from build123d import *

# Parameters (mm, degrees)
F0_R     = 3.175
F1_DEPTH = 3.048


with BuildPart() as f1:
    # F0 (on Front) → F1 (new body)
    with BuildSketch(Plane.XZ):
        with BuildLine():
            ThreePointArc((9.4772553384, -0.9525), (9.5130563464, -0.4768479324), (9.525, 0))
            ThreePointArc((9.525, 0), (6.8544082857, 6.6138273378), (0.3401785714, 9.5189234444))
            ThreePointArc((0.3401785714, 9.5189234444), (-6.948684782, 6.5147068085), (-9.4772553384, -0.9525))
            ThreePointArc((-9.4772553384, -0.9525), (-6.2623833552, -7.1769199322), (0.3401786416, -9.5189234418))
            ThreePointArc((0.3401786416, -9.5189234418), (6.5147068341, -6.948684758), (9.4772553384, -0.9525))
        make_face()
        Circle(F0_R, mode=Mode.SUBTRACT)
        with BuildLine():
            ThreePointArc((0.3401785714, 9.5189234444), (6.8544082857, 6.6138273378), (9.525, 0))
            ThreePointArc((9.525, 0), (9.5130563464, -0.4768479324), (9.4772553384, -0.9525))
            Line((9.4772553384, -0.9525), (10.4932062399, 9.1560838367))
            Line((10.4932062399, 9.1560838367), (0.3401785714, 9.5189234444))
        make_face()
        with BuildLine():
            ThreePointArc((-9.4772553384, -0.9525), (-6.948684782, 6.5147068085), (0.3401785714, 9.5189234444))
            Line((0.3401785714, 9.5189234444), (10.4932062399, 9.1560838367))
            Line((10.4932062399, 9.1560838367), (15.7954255641, 61.9125))
            ThreePointArc((15.7954255641, 61.9125), (0, 47.625), (-15.7954255641, 61.9125))
            Line((-15.7954255641, 61.9125), (-9.4772553384, -0.9525))
        make_face()
        Polygon((4.1081828244, 15.4546830389), (2.8649913232, 15.4546830389), (1.5788532065, 18.7389689503), (-2.5598443184, 18.7389689503), (-3.8301599978, 15.4546830389), (-5.0462273207, 15.4546830389), (-0.9640385005, 25.825160507), (0.0463371378, 25.825160507), align=None, mode=Mode.SUBTRACT)
        Polygon((4.1081828244, 35.1287536323), (2.8649913232, 35.1287536323), (1.5788532065, 38.4130395436), (-2.5598443184, 38.4130395436), (-3.8301599978, 35.1287536323), (-5.0462273207, 35.1287536323), (-0.9640385005, 45.4992311004), (0.0463371378, 45.4992311004), align=None, mode=Mode.SUBTRACT)
        with BuildLine():
            Line((10.4932062399, 9.1560838367), (9.4772553384, -0.9525))
            ThreePointArc((9.4772553384, -0.9525), (6.5147068341, -6.948684758), (0.3401786416, -9.5189234418))
            Line((0.3401786416, -9.5189234418), (44.7334821429, -7.9324362036))
            ThreePointArc((44.7334821429, -7.9324362036), (36.5125, 0), (44.7334821429, 7.9324362036))
            Line((44.7334821429, 7.9324362036), (10.4932062399, 9.1560838367))
        make_face()
        with BuildLine():
            ThreePointArc((-15.7504882737, 65.484375), (-15.8737438155, 63.6997054867), (-15.7954255641, 61.9125))
            ThreePointArc((-15.7954255641, 61.9125), (0, 47.625), (15.7954255641, 61.9125))
            ThreePointArc((15.7954255641, 61.9125), (15.8550939106, 62.7052534459), (15.875, 63.5))
            ThreePointArc((15.875, 63.5), (15.8438414904, 64.4941387366), (15.7504882737, 65.484375))
            ThreePointArc((15.7504882737, 65.484375), (0, 79.375), (-15.7504882737, 65.484375))
        make_face()
        with Locations((0, 63.5)):
            Circle(F0_R, mode=Mode.SUBTRACT)
        with BuildLine():
            ThreePointArc((52.3875, 0), (50.1620069047, 5.5115227815), (44.7334821429, 7.9324362036))
            ThreePointArc((44.7334821429, 7.9324362036), (36.5125, 0), (44.7334821429, -7.9324362036))
            ThreePointArc((44.7334821429, -7.9324362036), (50.1620069047, -5.5115227815), (52.3875, 0))
        make_face()
        with Locations((44.45, 0)):
            Circle(F0_R, mode=Mode.SUBTRACT)
        with BuildLine():
            Line((-9.4502929642, 115.490625), (-15.7504882737, 65.484375))
            ThreePointArc((-15.7504882737, 65.484375), (0, 79.375), (15.7504882737, 65.484375))
            Line((15.7504882737, 65.484375), (9.4502929642, 115.490625))
            ThreePointArc((9.4502929642, 115.490625), (9.5063048942, 114.896483242), (9.525, 114.3))
            ThreePointArc((9.525, 114.3), (-0.596483242, 104.7936951058), (-9.4502929642, 115.490625))
        make_face()
        with Locations((-3.175, 100.0252)):
            Circle(F0_R, mode=Mode.SUBTRACT)
        with BuildLine():
            ThreePointArc((9.4502929642, 115.490625), (0, 123.825), (-9.4502929642, 115.490625))
            ThreePointArc((-9.4502929642, 115.490625), (-0.596483242, 104.7936951058), (9.525, 114.3))
            ThreePointArc((9.525, 114.3), (9.5063048942, 114.896483242), (9.4502929642, 115.490625))
        make_face()
        with Locations((0, 114.3)):
            Circle(F0_R, mode=Mode.SUBTRACT)
    extrude(amount=F1_DEPTH)


solid = f1.part
The model under review builds one solid part; all positions refer to its coordinate system, in mm. A direction names the side the tool comes from. Give positions to 0.01 mm unless a question says otherwise; leave off trailing zeros. Loops run counter-clockwise (first coordinate to the right, second up) from the corner with the lowest first, then second, coordinate; pieces in that order, holes last. Notation, with made-up numbers: (57.25, 51) -> (102.25, 51) arc R25 cw to (102.25, 83) -> close; hole circle Ø10 at (-21, 65). An arc over 180 degrees is marked (long way). Write each question's results on one line, items separated by ' | '.
1) Draft analysis for pull direction Z (two halves, no side actions). For faces 4 (the face through (-12.556, -1.503, 90.838)), 5 (the face through (2.231, -1.503, 17.074)), 6 (the face through (3, 0, 43)), 7 (the face through (-15.873, -1.503, 63.725)), state which applies: pulls with the +Z half, pulls with the -Z half, needs draft (parallel to the pull), parting line crosses it, or undercut.
Conclusion:
face 4: pulls with the +Z half | face 5: undercut | face 6: needs draft | face 7: parting line crosses it
2) Take a section at A-A, the plane y = -2.4. Count the separate pieces of the cut face and the enclosed holes in it, plus the area to 3 significant figures.
Conclusion:
separate pieces: 1 | enclosed holes: 7 | area: 3,690 mm^2
3) Take a section at B-B, the plane x = 12.5. Give the boundary of the cut face in (y, z).
Conclusion:
outline: (-3.05, -9.08) -> (0, -9.08) -> (0, 9.08) -> (-3.05, 9.08) -> close; (-3.05, 29.12) -> (0, 29.12) -> (0, 91.28) -> (-3.05, 91.28) -> close
4) Tool access review of faces 1 (the face through (-3.186, -1.503, 36.794)), 2 (the face through (12.644, -1.503, 90.137)), 3 (the face through (13.107, -1.503, 35.165)): name each direction out of +Z, -Z, +X, -X, +Y, -Y from which nothing blocks a thin tool from reaching the whole face with its end or side.
Conclusion:
face 1: +Y, -Y | face 2: +Z, +X, +Y, -Y | face 3: +X, +Y, -Y
5) Insertion check: pin 1 Ø1.3 at (x, y) = (-4.5, -1) entering from +Z; pin 2 Ø1.5 at (x, y) = (27.5, -2.5) entering from +Z; pin 3 Ø0.9 at (x, y) = (-1, -1.5) entering from +Z. Each pin has a flat end and moves straight along its axis. Give the tip position at first contact, or say it passes through.
Conclusion:
pin 1: stops at z = 123.01 | pin 2: stops at z = 8.58 | pin 3: stops at z = 123.81
6) For line 1 along X through (y, z) = (-1.7, 37); line 2 along X through (y, z) = (-1.5, 62); line 3 along X through (y, z) = (-1.4, 67), list the stretches that pass through material, from the lowest coordinate up. Write a range as from..to.
Conclusion:
line 1: x = -13.29..-4.31, -3.11..2.13, 3.38..13.29 | line 2: x = -15.8..-2.8, 2.8..15.8 | line 3: x = -15.56..15.56
7) Take a section at D-D, the plane x = 40. Give the boundary of the cut face in (y, z), plus the area to 3 significant figures.
Conclusion:
outline: (-3.05, -8.1) -> (0, -8.1) -> (0, 8.1) -> (-3.05, 8.1) -> close | area: 49.4 mm^2
8) Take a section at C-C, the plane z = 106.5. Give the boundary of the cut face in (x, y).
Conclusion:
outline: (-10.58, -3.05) -> (10.58, -3.05) -> (10.58, 0) -> (-10.58, 0) -> close
